from build123d import *

# Parameters (mm, degrees)
F0_R        = 8
F1_DEPTH    = 10
F3_DEPTH    = 10
F5_D        = 2
F5_DEPTH    = 8.001
F6_D        = 2
F7_T1_DEPTH = 37.4894960018
F9_DEPTH    = 8
F11_D       = 2
F11_DEPTH   = 8.0010001
F13_D       = 2
F14_R       = 1.99999


# Not quite as in the source:
# - a fillet or chamfer that OpenCascade refuses, or shapes differently, is made with other operations: its cross-section is extruded or revolved along the edge and cut away or added
# - a fillet or chamfer is up to 0.001 mm smaller than in the source, because OpenCascade refuses the exact size


with BuildPart() as f1:
    # F0 (on Top) → F1 (new body, symmetric)
    with BuildSketch(Plane.XY):
        Circle(F0_R)
    extrude(amount=F1_DEPTH, both=True)

    # F2 (on face) → F3 (cut)
    with BuildSketch(Plane.XY.offset(10)):
        with BuildLine():
            ThreePointArc((5, 6.2449979984), (0, 8), (-5, 6.2449979984))
            Line((-5, 6.2449979984), (-5, -6.2449979984))
            ThreePointArc((-5, -6.2449979984), (0, -8), (5, -6.2449979984))
            Line((5, -6.2449979984), (5, 6.2449979984))
        make_face()
    extrude(amount=-F3_DEPTH, mode=Mode.SUBTRACT)

    # F5 (through all, one way)
    with BuildSketch(Plane.YZ):
        with Locations((0, 6)):
            Circle(F5_D / 2)
    extrude(amount=-F5_DEPTH, mode=Mode.SUBTRACT)

    # F6 (through all)
    with Locations(Plane(origin=(0, 0, 0), x_dir=(0, 1, 0), z_dir=(-1, 0, 0))):
        with Locations((0, -6)):
            Hole(F6_D / 2)

    # F7: fillet of radius 5 on 2 edges, made by hand

    # F7_s2 → F7_t1 (cut)
    with BuildSketch(Plane.XZ.offset(-18.7447480009)):
        with BuildLine():
            ThreePointArc((-4.9999, 5.0001), (-6.4643660941, 8.5356339059), (-9.9999, 10.0001))
            Line((-9.9999, 10.0001), (-9.9999, 10.1001))
            ThreePointArc((-9.9999, 10.1001), (-7.49995, 10.1), (-5, 10.1))
            Line((-5, 10.1), (-4.9, 10))
            ThreePointArc((-4.9, 10), (-4.9, 7.50005), (-4.8999, 5.0001))
            Line((-4.8999, 5.0001), (-4.9999, 5.0001))
        make_face()
        with BuildLine():
            ThreePointArc((9.9999, 10.0001), (6.4643660941, 8.5356339059), (4.9999, 5.0001))
            Line((4.9999, 5.0001), (4.8999, 5.0001))
            ThreePointArc((4.8999, 5.0001), (4.9, 7.50005), (4.9, 10))
            Line((4.9, 10), (5, 10.1))
            ThreePointArc((5, 10.1), (7.49995, 10.1), (9.9999, 10.1001))
            Line((9.9999, 10.1001), (9.9999, 10.0001))
        make_face()
    extrude(amount=F7_T1_DEPTH, mode=Mode.SUBTRACT)

    # F8 (on face) → F9 (cut)
    with BuildSketch(Plane(origin=(0, 0, -10), x_dir=(1, 0, 0), z_dir=(0, 0, -1))):
        with BuildLine():
            Line((7.7459666924, 2), (-7.7459666924, 2))
            ThreePointArc((-7.7459666924, 2), (-8, 0), (-7.7459666924, -2))
            Line((-7.7459666924, -2), (7.7459666924, -2))
            ThreePointArc((7.7459666924, -2), (7.9362375701, -1.0080343399), (8, 0))
            ThreePointArc((8, 0), (7.9362375701, 1.0080343399), (7.7459666924, 2))
        make_face()
    extrude(amount=-F9_DEPTH, mode=Mode.SUBTRACT)

    # F11 (through all, one way)
    with BuildSketch(Plane.XZ):
        with Locations((0, -7)):
            Circle(F11_D / 2)
    extrude(amount=-F11_DEPTH, mode=Mode.SUBTRACT)

    # F13 (through all)
    with Locations(Plane(origin=(0, 0, 0), x_dir=(1, 0, 0), z_dir=(0, 1, 0))):
        with Locations((0, 7)):
            Hole(F13_D / 2)

    # F14 (radius 2 in the source; OpenCascade refuses exactly that, so slightly less here)
    f14_edges = [f1.edges().sort_by_distance(p)[0] for p in [
        (0, -2, -10),
        (0, 2, -10),
    ]]
    fillet(f14_edges, radius=F14_R)


solid = f1.part
Could you check a few things on this model? Use its own coordinates, in mm. A direction names the side the tool comes from. Give positions to 0.01 mm unless a question says otherwise; leave off trailing zeros. Order: outer loops, then holes, each group sorted by start corner. A loop starts at its lowest first (then second) coordinate and runs counter-clockwise, first axis right, second up.
1. Suppose I cut it at B-B (z = -7). List the corners of the cut face in (x, y) for me, plus the area to 3 significant figures.
2. Suppose I cut it at D-D (x = 5.75). List the corners of the cut face in (y, z) for me, plus the area to 3 significant figures.
3. Suppose I cut it at A-A (x = 0). Give the number of separate pieces and of enclosed holes in the cut face, plus the area to 3 significant figures.
4. Suppose I cut it at C-C (y = -6). List the corners of the cut face in (x, z) for me, plus the area to 3 significant figures.
5. For faces 5 (the cylindrical face through (0.11, 2.6, -9.43)), 6 (the flat face through (0, 0, 0)), 7 (the cylindrical face through (-6, 0, 5)), which set-ups out of +Z, -Z, +X, -X, +Y, -Y let a thin tool reach every point of the face, with its end or its side?
6. We'd pull the mould along Y, two halves only. Please class faces 1 (the cylindrical face through (-0.11, -2.6, -9.43)), 2 (the cylindrical face through (0, -5, -8)), 3 (the cylindrical face through (7.39, -3.06, -2.25)), 4 (the flat face through (0, 0, -2)): pulls with the +Y half, pulls with the -Y half, needs draft (parallel to the pull), parting line crosses it, or undercut.
7. Will these pins go through, and if not, where does the flat tip stop? P1, Ø5.5, axis at y = 2.5, z = 3.5, coming from the +X side; P2, Ø8, axis at x = -2, y = 3, coming from the +Z side; P3, Ø6, axis at x = 1, z = 4.5, coming from the -Y side; P4, Ø8, axis at y = -6.5, z = -2.5, coming from the +X side.
8. I need wall thicknesses on L1, parallel to Y at x = -4, z = -4.75; L2, parallel to X at y = 0, z = 2; L3, parallel to X at y = -5.25, z = 7.75. Which ranges of each line are inside material? Lowest first, please.
Solved:
1. outline: (-7.75, -2) arc R8 ccw to (-1, -7.94) - (-1, -2) - close; (-7.75, 2) - (-1, 2) - (-1, 7.94) arc R8 ccw to start; (1, -7.94) arc R8 ccw to (7.75, -2) - (1, -2) - close; (1, 2) - (7.75, 2) arc R8 ccw to (1, 7.94) - close
1. area: 114 mm2
2. outline: (-5.56, -10) - (-4, -10) arc R2 ccw to (-2, -8) - (-2, -2) - (2, -2) - (2, -8) arc R2 ccw to (4, -10) - (5.56, -10) - (5.56, 7.63) - (-5.56, 7.63) - close; hole circle Ø2 at (0, 6)
2. area: 159 mm2
3. separate pieces: 3
3. enclosed holes: 0
3. area: 102 mm2
4. outline: (-5.29, -10) - (5.29, -10) - (5.29, 6.68) arc R5 ccw to (5, 5.03) - (5, 0) - (-5, 0) - (-5, 5.03) arc R5 ccw to (-5.29, 6.68) - close; hole circle Ø2 at (0, -7)
4. area: 106 mm2
5. face 5: -Z, +X, -X
5. face 6: +Z, +Y, -Y
5. face 7: +X, -X
6. face 1: undercut
6. face 2: needs draft
6. face 3: parting line crosses it
6. face 4: undercut
7. P1: stops at x = 8
7. P2: stops at z = 8
7. P3: passes through
7. P4: stops at x = 7.6
8. L1: y = -6.93 to -2, 2 to 6.93
8. L2: x = -8 to -5, 5 to 8
8. L3: x = -6.04 to -5.82, 5.82 to 6.04
